Can you work these out from the drawing? Everything is in mm from the part's minimum corner. Coordinates: 2 decimals unless noted, no trailing zeros. Write each loop counter-clockwise with the first axis right and the second up, starting at its lowest first coordinate (ties: lowest second). Pieces come first, ordered by that corner, then holes.
(1) For pin 1 Ø12 at (x, z) = (27, 2124) entering from -Y; pin 2 Ø6 at (y, z) = (82.5, 1212.5) entering from +X; pin 3 Ø10 at (x, z) = (26, 2103) entering from +Y, each with a flat end and sliding along its axis, tell me the tip position at first contact or that it passes through.
(2) Imagine slicing it at C-C, the plane z = 1255.5. List the corners of the cut face in (x, y) for me, plus the area to 3 significant figures.
(3) Please list where these lines run through material, in increasing order: probe 1 along Z at (x, y) = (12, 89); probe 2 along Z at (x, y) = (54.5, 120); probe 3 along X at (y, z) = (77, 890).
(4) Imagine slicing it at A-A, the plane y = 76.2. List the corners of the cut face in (x, z) for me, plus the area to 3 significant figures.
(5) Imagine slicing it at B-B, the plane x = 38.1. List the corners of the cut face in (y, z) for me.
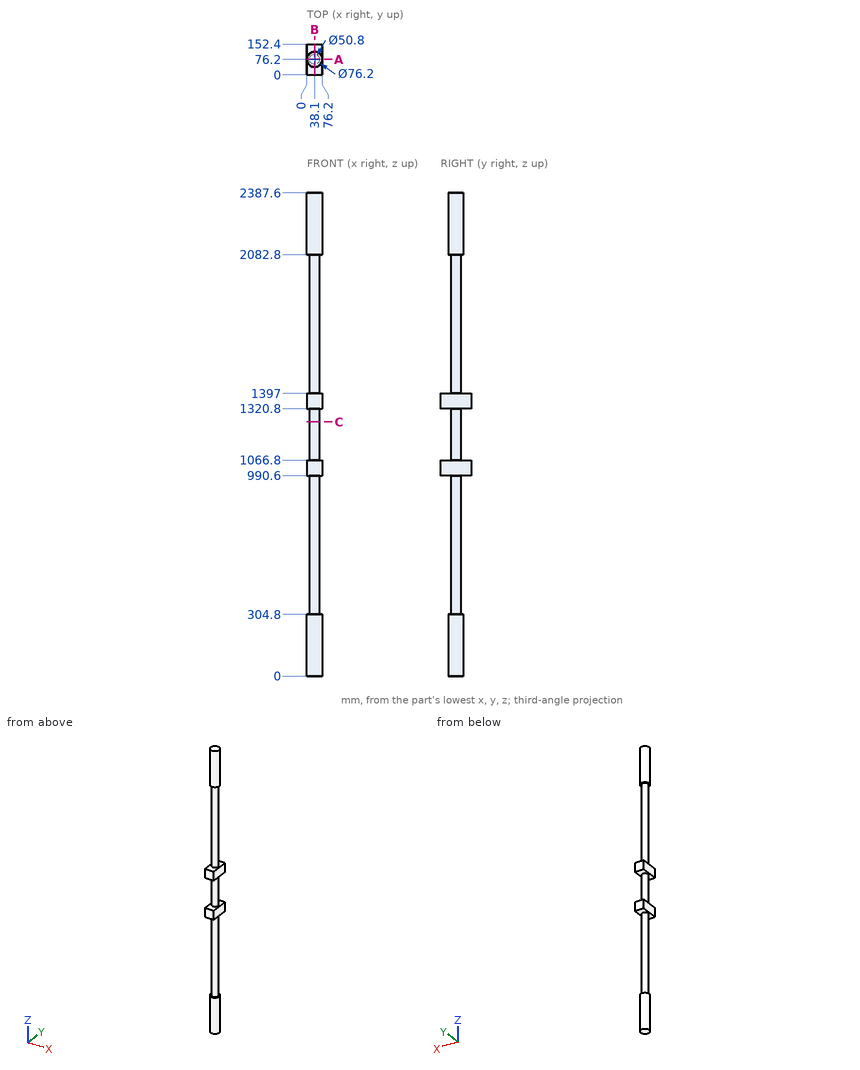
Recorded:
1. pin 1: stops at y = 38.44
1. pin 2: stops at x = 63.28
1. pin 3: stops at y = 113.63
2. outline: circle Ø50.8 at (38.1, 76.2)
2. area: 2,030 mm2
3. probe 1: z = 0 to 304.8, 990.6 to 1066.8, 1320.8 to 1397, 2082.8 to 2387.6
3. probe 2: z = 990.6 to 1066.8, 1320.8 to 1397
3. probe 3: x = 12.71 to 63.49
4. outline: (0, 0) - (76.2, 0) - (76.2, 304.8) - (63.5, 304.8) - (63.5, 990.6) - (76.2, 990.6) - (76.2, 1066.8) - (63.5, 1066.8) - (63.5, 1320.8) - (76.2, 1320.8) - (76.2, 1397) - (63.5, 1397) - (63.5, 2082.8) - (76.2, 2082.8) - (76.2, 2387.6) - (0, 2387.6) - (0, 2082.8) - (12.7, 2082.8) - (12.7, 1397) - (0, 1397) - (0, 1320.8) - (12.7, 1320.8) - (12.7, 1066.8) - (0, 1066.8) - (0, 990.6) - (12.7, 990.6) - (12.7, 304.8) - (0, 304.8) - close
4. area: 141,000 mm2
5. outline: (0, 990.6) - (50.8, 990.6) - (50.8, 304.8) - (38.1, 304.8) - (38.1, 0) - (114.3, 0) - (114.3, 304.8) - (101.6, 304.8) - (101.6, 990.6) - (152.4, 990.6) - (152.4, 1066.8) - (101.6, 1066.8) - (101.6, 1320.8) - (152.4, 1320.8) - (152.4, 1397) - (101.6, 1397) - (101.6, 2082.8) - (114.3, 2082.8) - (114.3, 2387.6) - (38.1, 2387.6) - (38.1, 2082.8) - (50.8, 2082.8) - (50.8, 1397) - (0, 1397) - (0, 1320.8) - (50.8, 1320.8) - (50.8, 1066.8) - (0, 1066.8) - close
